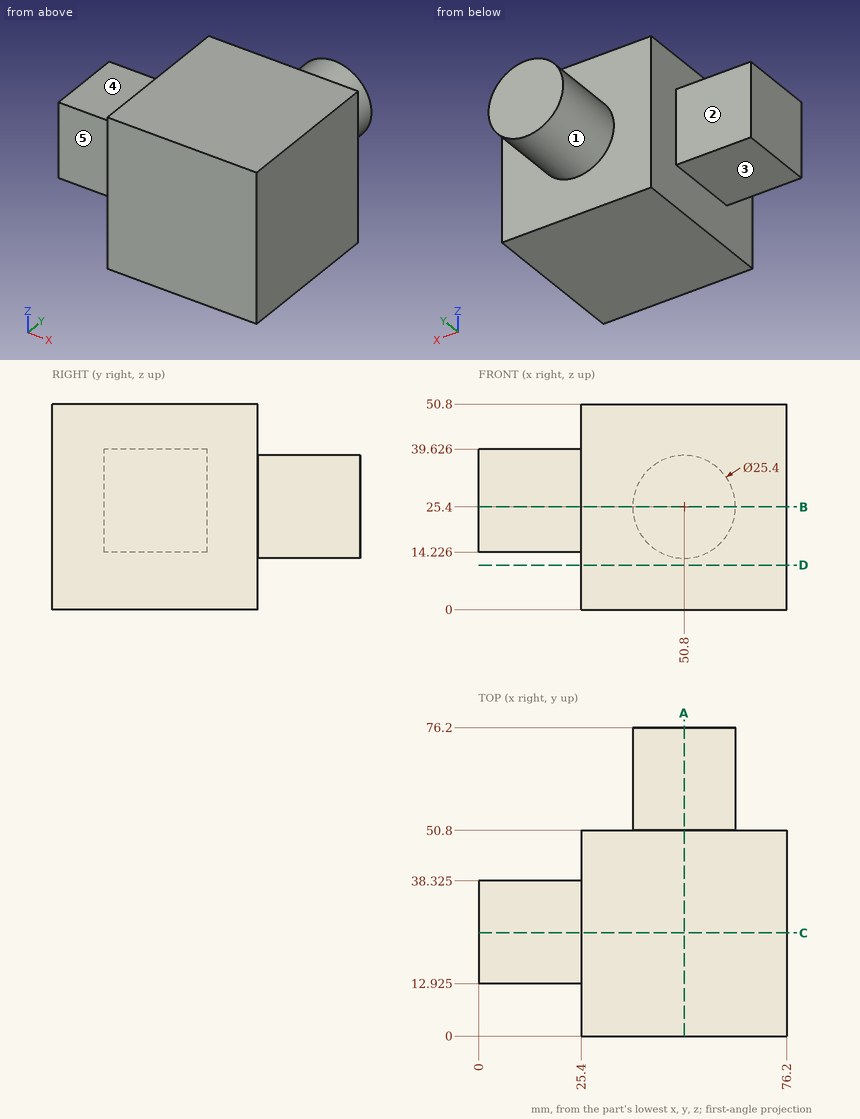
Print and shaded views of the part. All mm, measured from the part's lowest x, y and z. A direction names the side the tool comes from. Give positions to 0.01 mm unless a question says otherwise; leave off trailing zeros. Write each loop counter-clockwise with the first axis right and the second up, starting at its lowest first coordinate (ties: lowest second). Pieces come first, ordered by that corner, then holes. Notation, with made-up numbers: (-29, 70.5) -> (12, 70.5) arc R22 ccw to (12, 92.5) -> close; hole circle Ø11 at (20, 9). An arc over 180 degrees is marked (long way). Use CSV: the item, a comma, the result in double quotes. Start each with the question number.
1) Pin check, flat tips, straight feed: P1, Ø8, axis at y = 44, z = 40, coming from the -X side; P2, Ø6, axis at y = 59.5, z = 20, coming from the +X side; P3, Ø20.5, axis at x = 12.5, z = 32.5, coming from the +Y side (1 decimal); P4, Ø12, axis at y = 26, z = 44.5, coming from the -X side. Stop position of each tip, or through.
2) Cut at C-C on y = 25.5. List the corners of the cut face in (x, z).
3) Drill centre lines: L1, parallel to X at y = 39, z = 25.5; L2, parallel to Y at x = 62, z = 36; L3, parallel to Z at x = 4, y = 21. Where is each one in solid material? Low to high.
4) Tool access for the marked faces 1, 2, 3, 4 and 5: list every direction of +Z, -Z, +X, -X, +Y, -Y with a clear straight run to the whole face (end or side of a thin tool).
5) Cut at A-A on x = 50.8. List the corners of the cut face in (y, z), plus the area to 3 significant figures.
6) Cut at B-B on z = 25.4. List the corners of the cut face in (x, y) (1 decimal), plus the area to 3 significant figures.
7) Cut at D-D on z = 11. List the corners of the cut face in (x, y).
Final values:
1,P1,"stops at x = 25.4"
1,P2,"stops at x = 63.27"
1,P3,"stops at y = 38.3"
1,P4,"stops at x = 0"
2,outline,"(0, 14.23) -> (25.4, 14.23) -> (25.4, 0) -> (76.2, 0) -> (76.2, 50.8) -> (25.4, 50.8) -> (25.4, 39.63) -> (0, 39.63) -> close"
3,L1,"x = 25.4 to 76.2"
3,L2,"y = 0 to 50.8"
3,L3,"z = 14.23 to 39.63"
4,face 1,"+Y"
4,face 2,"+Z, -Z, -X, +Y"
4,face 3,"-Z, -X, +Y, -Y"
4,face 4,"+Z, -X, +Y, -Y"
4,face 5,"+Z, -Z, -X, -Y"
5,outline,"(0, 0) -> (50.8, 0) -> (50.8, 12.7) -> (76.2, 12.7) -> (76.2, 38.1) -> (50.8, 38.1) -> (50.8, 50.8) -> (0, 50.8) -> close"
5,area,"3,230 mm2"
6,outline,"(0, 12.9) -> (25.4, 12.9) -> (25.4, 0) -> (76.2, 0) -> (76.2, 50.8) -> (63.5, 50.8) -> (63.5, 76.2) -> (38.1, 76.2) -> (38.1, 50.8) -> (25.4, 50.8) -> (25.4, 38.3) -> (0, 38.3) -> close"
6,area,"3,870 mm2"
7,outline,"(25.4, 0) -> (76.2, 0) -> (76.2, 50.8) -> (25.4, 50.8) -> close"
